Model file for the job. Use its own axes, mm. A direction names the side the tool comes from. Round coordinates to 2 decimals unless told otherwise and drop trailing zeros. Order: outer loops, then holes, each group sorted by start corner. A loop starts at its lowest first (then second) coordinate and runs counter-clockwise, first axis right, second up. Notation, with made-up numbers: (84, 32.5) - (143, 32.5) arc R20 ccw to (143, 39.5) - close; hole circle Ø7 at (14, 60.25). An arc over 180 degrees is marked (long way). Answer as CSV lines item,"result". Start each with the question number.
1. Pull direction X, two halves, no side cores. Call faces 6 (the face through (21, 3.5, -4.2)), 7 (the face through (-16.44, 2.52, -4.17)), 8 (the face through (0.1, 2.5, 9.1)): released by +X, released by -X, zero draft, split by the parting line, or undercut.
2. Wall check: line 1 along X through (y, z) = (2.95, 12.1); line 2 along Z through (x, y) = (-2, 2.7); line 3 along Z through (x, y) = (12, 3). Give the ranges that are in metal, low to high. Write a range as [from, to].
3. 3-axis set-ups, long thin cutter, end or side, ignore diameter. For faces 1 (the face through (-9.3, 1, -10.8)), 2 (the face through (-11, 2, -16.1)), 3 (the face through (16.56, 1.52, -4.17)), 4 (the face through (11, 2, 8.1)), 5 (the face through (0, 2, -8.1)): which of +Z, -Z, +X, -X, +Y, -Y reach the whole face in a straight line?
4. Band-saw the part on A-A on x = 0. List the corners of the cut face in (y, z), then the cut area to 3 significant figures.
5. Band-saw the part on D-D on z = -12.1. List the corners of the cut face in (x, y).
6. Band-saw the part on C-C on y = 1.75. List the corners of the cut face in (x, z), then the cut area to 3 significant figures.
7. Band-saw the part on B-B on z = 12.1. List the corners of the cut face in (x, y), then the cut area to 3 significant figures.
8. Pin check, flat tips, straight feed: pin 1 Ø4 at (x, z) = (0, 12.1) entering from +Y; pin 2 Ø2 at (x, y) = (10.5, 2.5) entering from +Z; pin 3 Ø1.2 at (y, z) = (2, 12) entering from -X. Stop position of each tip, or through.
```python
from build123d import *

# Parameters (mm, degrees)
EXTRUDE_1_DEPTH     = 4
SKETCH_2_R          = 1.5
CUT_EXTRUDE_2_DEPTH = 27.762100067
SKETCH_3_R          = 3
CUT_EXTRUDE_3_DEPTH = 3
CUT_EXTRUDE_4_DEPTH = 39.65022639
FILLET_1_R          = 1


with BuildPart() as part:
    # 草图1 → 凸台-拉伸1 (new body)
    with BuildSketch(Plane(origin=(0, 0, 0), x_dir=(1, 0, 0), z_dir=(0, 1, 0))):
        Polygon((-21, 16.1), (-4.1, 16.1), (-4.1, 8.1), (4.1, 8.1), (4.1, 16.1), (21, 16.1), (21, -8.1), (3.9, -8.1), (3.9, -16.1), (-3.9, -16.1), (-3.9, -8.1), (-21, -8.1), align=None)
    extrude(amount=EXTRUDE_1_DEPTH)

    # 草图2 → 切除-拉伸2 (cut, through all)
    with BuildSketch(Plane(origin=(0, 0, 0), x_dir=(1, 0, 0), z_dir=(0, 1, 0))):
        with Locations(Location((-8, 12.1, 0), (0, 0, 270))):
            Circle(SKETCH_2_R)
        with Locations(Location((8, 12.1, 0), (0, 0, 270))):
            Circle(SKETCH_2_R)
        with Locations(Location((0, -12.1, 0), (0, 0, 270))):
            Circle(SKETCH_2_R)
    extrude(amount=CUT_EXTRUDE_2_DEPTH, mode=Mode.SUBTRACT)

    # 草图3 → 切除-拉伸3 (cut)
    with BuildSketch(Plane(origin=(0, 4, 0), x_dir=(1, 0, 0), z_dir=(0, 1, 0))):
        with Locations(Location((-8, 12.1, 0), (0, 0, 270))):
            Circle(SKETCH_3_R)
        with Locations(Location((8, 12.1, 0), (0, 0, 270))):
            Circle(SKETCH_3_R)
        with Locations(Location((0, -12.1, 0), (0, 0, 270))):
            Circle(SKETCH_3_R)
    extrude(amount=-CUT_EXTRUDE_3_DEPTH, mode=Mode.SUBTRACT)

    # 草图4 → 切除-拉伸4 (cut, through all)
    with BuildSketch(Plane(origin=(0, 0, -16.1), x_dir=(-1, 0, 0), z_dir=(0, 0, -1))):
        Polygon((-21, 3), (-12, 0), (-21, 0), align=None)
        Polygon((12, 4), (21, 1), (21, 4), align=None)
    extrude(amount=-CUT_EXTRUDE_4_DEPTH, mode=Mode.SUBTRACT)

    # 圆角1
    fillet_1_edges = [part.edges().sort_by_distance(p)[0] for p in [
        (3.9, 2, 16.1),
        (-3.9, 2, 16.1),
    ]]
    fillet(fillet_1_edges, radius=FILLET_1_R)


solid = part.part
```
Reply:
1,face 6,"released by +X"
1,face 7,"released by -X"
1,face 8,"undercut"
2,line 1,"x = [-3.9, -3], [3, 3.9]"
2,line 2,"z = [-8.1, 9.86], [14.34, 16.1]"
2,line 3,"z = [-16.1, 8.1]"
3,face 1,"+Y"
3,face 2,"-Z, +X, -X, +Y, -Y"
3,face 3,"+Z, -Z, +X, -Y"
3,face 4,"+Z, +X, +Y, -Y"
3,face 5,"-Z, +Y, -Y"
4,outline,"(0, -8.1) - (4, -8.1) - (4, 9.1) - (1, 9.1) - (1, 10.6) - (0, 10.6) - close; (0, 13.6) - (1, 13.6) - (1, 15.1) - (4, 15.1) - (4, 16.1) - (0, 16.1) - close"
4,area,"75.8 mm2"
5,outline,"(-21, 0) - (-9.5, 0) - (-9.5, 1) - (-11, 1) - (-11, 4) - (-12, 4) - (-21, 1) - close; (-6.5, 0) - (-4.1, 0) - (-4.1, 4) - (-5, 4) - (-5, 1) - (-6.5, 1) - close; (4.1, 0) - (6.5, 0) - (6.5, 1) - (5, 1) - (5, 4) - (4.1, 4) - close; (9.5, 0) - (12, 0) - (21, 3) - (21, 4) - (11, 4) - (11, 1) - (9.5, 1) - close"
6,outline,"(-18.75, -16.1) - (-4.1, -16.1) - (-4.1, -8.1) - (4.1, -8.1) - (4.1, -16.1) - (17.25, -16.1) - (17.25, 8.1) - (3.9, 8.1) - (3.9, 15.1) arc R1 ccw to (2.9, 16.1) - (-2.9, 16.1) arc R1 ccw to (-3.9, 15.1) - (-3.9, 8.1) - (-18.75, 8.1) - close; hole circle Ø6 at (-8, -12.1); hole circle Ø6 at (0, 12.1); hole circle Ø6 at (8, -12.1)"
6,area,"783 mm2"
7,outline,"(-3.9, 0) - (-1.5, 0) - (-1.5, 1) - (-3, 1) - (-3, 4) - (-3.9, 4) - close; (1.5, 0) - (3.9, 0) - (3.9, 4) - (3, 4) - (3, 1) - (1.5, 1) - close"
7,area,"10.2 mm2"
8,pin 1,"stops at y = 1"
8,pin 2,"stops at z = 8.1"
8,pin 3,"stops at x = -3.9"
